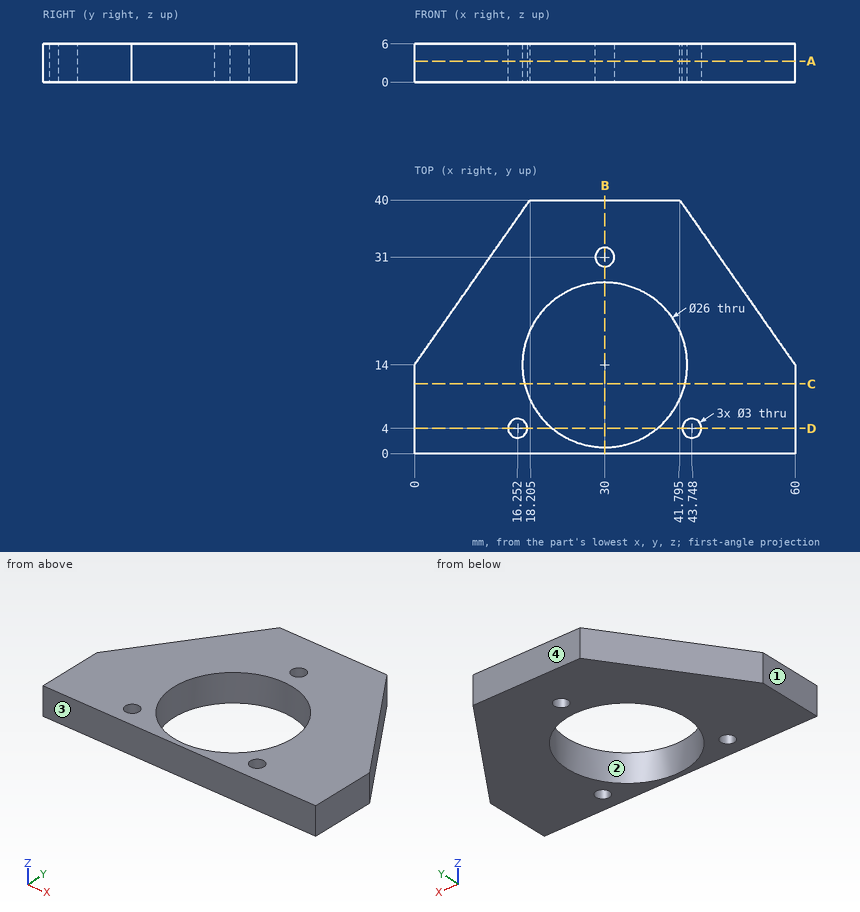
The figure shows three views and two pictorial views of one solid part (mm, origin at its lowest corner). Answer the questions. Give positions to 0.01 mm unless a question says otherwise; leave off trailing zeros. Order: outer loops, then holes, each group sorted by start corner. A loop starts at its lowest first (then second) coordinate and runs counter-clockwise, first axis right, second up. Notation, with made-up numbers: (-3, -9.75) -> (32, -9.75) arc R21 ccw to (32, 12.25) -> close; hole circle Ø2 at (9.25, 8). An arc over 180 degrees is marked (long way). Write each question's results on one line, items separated by ' | '.
Q1. Straight lines are drawn through the part: probe 1 along Y at (x, z) = (30, 4.65); probe 2 along Y at (x, z) = (19, 1.55) (1 decimal); probe 3 along Y at (x, z) = (21, 5.2). For each, find the intervals that lie inside material, in ascending order. Write a range as from..to.
Checked values:
probe 1: y = 0..1, 27..29.5, 32.5..40 | probe 2: y = 0..7.1, 20.9..40 | probe 3: y = 0..4.62, 23.38..40
Q2. The part is cut by section D-D, the plane y = 4. Give the vertices of the cut face in (x, z), and give its area (3 significant figures).
Checked values:
outline: (0, 0) -> (14.75, 0) -> (14.75, 6) -> (0, 6) -> close; (17.75, 0) -> (21.69, 0) -> (21.69, 6) -> (17.75, 6) -> close; (38.31, 0) -> (42.25, 0) -> (42.25, 6) -> (38.31, 6) -> close; (45.25, 0) -> (60, 0) -> (60, 6) -> (45.25, 6) -> close | area: 224 mm^2
Q3. The part is cut by section A-A, the plane z = 3.3. Give the vertices of the cut face in (x, y) (1 decimal), and give its area (3 significant figures).
Checked values:
outline: (0, 0) -> (60, 0) -> (60, 14) -> (41.8, 40) -> (18.2, 40) -> (0, 14) -> close; hole circle Ø3 at (16.3, 4); hole circle Ø26 at (30, 14); hole circle Ø3 at (30, 31); hole circle Ø3 at (43.7, 4) | area: 1,370 mm^2
Q4. The part is cut by section C-C, the plane y = 11. Give the vertices of the cut face in (x, z).
Checked values:
outline: (0, 0) -> (17.35, 0) -> (17.35, 6) -> (0, 6) -> close; (42.65, 0) -> (60, 0) -> (60, 6) -> (42.65, 6) -> close
Q5. This flat-tipped pin is pushed along its axis until it touches: P1, Ø8, axis at x = 14, y = 35, coming from the +Z side. Where does it stop, or does it pass through?
Checked values:
P1: stops at z = 6
Q6. Determine the mould class of the marked faces 1, 2, 3 and 4 for opening direction Y: pulls with the +Y half, pulls with the -Y half, needs draft (parallel to the pull), parting line crosses it, or undercut.
Checked values:
face 1: needs draft | face 2: undercut | face 3: pulls with the -Y half | face 4: pulls with the +Y half
Q7. The part is cut by section B-B, the plane x = 30. Give the vertices of the cut face in (y, z), and give its area (3 significant figures).
Checked values:
outline: (0, 0) -> (1, 0) -> (1, 6) -> (0, 6) -> close; (27, 0) -> (29.5, 0) -> (29.5, 6) -> (27, 6) -> close; (32.5, 0) -> (40, 0) -> (40, 6) -> (32.5, 6) -> close | area: 66.0 mm^2
